For this review, take the finished solid that the model builds, in its own axes (mm). Face numbers are marked on the shaded views. A direction names the side the tool comes from. Round coordinates to 2 decimals unless told otherwise and drop trailing zeros. Write each loop counter-clockwise with the first axis right and the second up, starting at its lowest first coordinate (ties: lowest second). Pieces come first, ordered by that corner, then holes. Notation, with made-up numbers: M 78.5,12 L 85.5,12 A33 cw 85.5,45 Z; hole C 17,23.5 d5. An arc over 180 degrees is marked long. Answer in a Markdown table with one row per item.
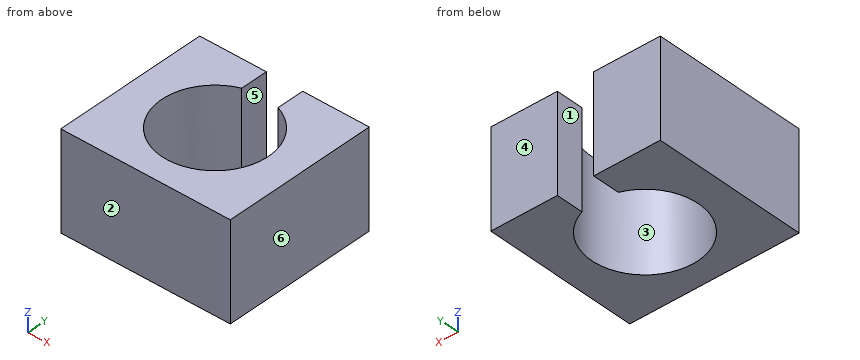
```python
from build123d import *

# Parameters (mm, degrees)
SKETCH_1_W          = 70
SKETCH_1_H          = 64
EXTRUDE_1_DEPTH     = 20
SKETCH_2_R          = 22
CUT_EXTRUDE_1_DEPTH = 40
SKETCH_3_W          = 15
SKETCH_3_H          = 40
CUT_EXTRUDE_2_DEPTH = 20


with BuildPart() as part:
    # 草图1 → 凸台-拉伸1 (new, symmetric)
    with BuildSketch(Plane.XY):
        Rectangle(SKETCH_1_W, SKETCH_1_H)
    extrude(amount=EXTRUDE_1_DEPTH, both=True)

    # 草图2 → 切除-拉伸1 (cut)
    with BuildSketch(Plane.XY.offset(20)):
        Circle(SKETCH_2_R)
    extrude(amount=-CUT_EXTRUDE_1_DEPTH, mode=Mode.SUBTRACT)

    # 草图3 → 切除-拉伸2 (cut)
    with BuildSketch(Plane(origin=(0, 32, 0), x_dir=(1, 0, 0), z_dir=(0, 1, 0))):
        Rectangle(SKETCH_3_W, SKETCH_3_H)
    extrude(amount=-CUT_EXTRUDE_2_DEPTH, mode=Mode.SUBTRACT)


solid = part.part
```
Q1. For probe 1 along X at (y, z) = (0, 1); probe 2 along X at (y, z) = (23.5, 12); probe 3 along Y at (x, z) = (0, -7.5), list the stretches that pass through material, from the lowest coordinate up.
Found:
| item | result |
|---|---|
| probe 1 | -35 to -22, 22 to 35 |
| probe 2 | -35 to -7.5, 7.5 to 35 |
| probe 3 | -32 to -22 |
Q2. Take a section at B-B (z = -1.5). State the section outline as (x, y) points, then the cut area to 3 significant figures.
Found:
| item | result |
|---|---|
| outline | M -35,-32 L 35,-32 L 35,32 L 7.5,32 L 7.5,20.68 A22 cw long -7.5,20.68 L -7.5,32 L -35,32 Z |
| area | 2,800 mm² |
Q3. Mouldability with a two-part tool opening along X and no side actions: class the marked faces 3, 4, 5 and 6 as +X half, -X half, draft (parallel to the pull), parting line (faces both ways), or undercut.
Found:
| item | result |
|---|---|
| face 3 | undercut |
| face 4 | draft |
| face 5 | undercut |
| face 6 | +X half |
Q4. Machinability: for the marked faces 1 and 2, which of the approach directions +Z, -Z, +X, -X, +Y, -Y give a long, thin tool a straight path to every point of the face, cutting with its end or side? Answer none if there is none.
Found:
| item | result |
|---|---|
| face 1 | +Z, -Z, +Y |
| face 2 | +Z, -Z, +X, -X, -Y |
Q5. Take a section at A-A (y = 0). State the section outline as (x, z) points, then the cut area to 3 significant figures.
Found:
| item | result |
|---|---|
| outline | M -35,-20 L -22,-20 L -22,20 L -35,20 Z; M 22,-20 L 35,-20 L 35,20 L 22,20 Z |
| area | 1,040 mm² |
Q6. Take a section at D-D (x = 0). State the section outline as (y, z) points, then the cut area to 3 significant figures.
Found:
| item | result |
|---|---|
| outline | M -32,-20 L -22,-20 L -22,20 L -32,20 Z |
| area | 400 mm² |
Q7. Take a section at C-C (y = 28). State the section outline as (x, z) points, then the cut area to 3 significant figures.
Found:
| item | result |
|---|---|
| outline | M -35,-20 L -7.5,-20 L -7.5,20 L -35,20 Z; M 7.5,-20 L 35,-20 L 35,20 L 7.5,20 Z |
| area | 2,200 mm² |
